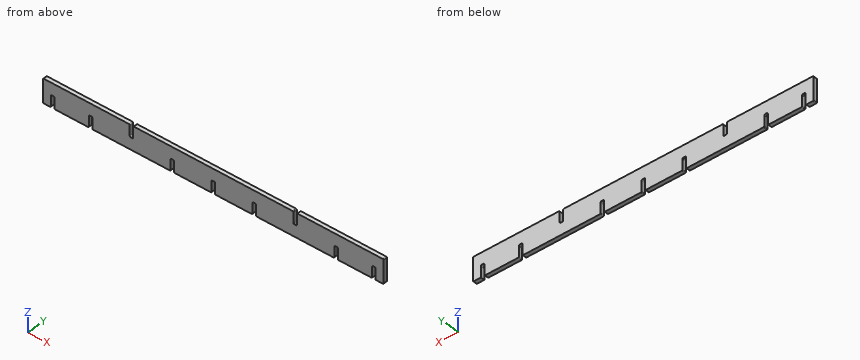
Autodesk Inventor part; units mm, degrees
ref_plane "YZ Plane" through (0, 0, 0) normal (1, 0, 0) x (0, 1, 0)
ref_plane "XZ Plane" through (0, 0, 0) normal (0, 1, 0) x (-1, 0, 0)
ref_plane "XY Plane" through (0, 0, 0) normal (0, 0, 1) x (1, 0, 0)
sketch "Sketch1" plane through (0, 0, 0) normal (0, 1, 0) x (-1, 0, 0)
  line L0 (0, 0) -> (435, 0)
  line L1 (435, 0) -> (435, -30)
  line L2 (435, -30) -> (0, -30)
  line L3 (0, -30) -> (0, 0)
  dimension "d0" = 435
  dimension "d1" = 30
extrude "Extrusion1" add sketch "Sketch1" along normal blind 5
sketch "Sketch2" plane through (0, 5, 0) normal (0, 1, 0) x (1, 0, 0)
  line L0 (0, 30) -> (-435, 30)
  line L1 (-435, 30) -> (-425, 30)
  line L2 (-425, 30) -> (-420.5, 30)
  line L3 (-420.5, 30) -> (-420.5, 15)
  line L4 (-420.5, 15) -> (-425, 15)
  line L5 (-425, 15) -> (-425, 30)
  line L6 (-420.5, 30) -> (-219.75, 30)
  line L7 (-219.75, 30) -> (-215.25, 30)
  line L8 (-215.25, 30) -> (-215.25, 15)
  line L9 (-215.25, 15) -> (-219.75, 15)
  line L10 (-219.75, 15) -> (-219.75, 30)
  line L11 (-215.25, 30) -> (-14.5, 30)
  line L12 (-14.5, 30) -> (-10, 30)
  line L13 (-10, 30) -> (-10, 15)
  line L14 (-10, 15) -> (-14.5, 15)
  line L15 (-14.5, 15) -> (-14.5, 30)
  point P0 (0, 0)
  dimension "d4" = 10
  dimension "d5" = 4.5
  dimension "d6" = 15
  dimension "d7" = 200.75
  dimension "d8" = 4.5
  dimension "d9" = 15
  dimension "d10" = 200.75
  dimension "d11" = 4.5
  dimension "d12" = 15
extrude "Extrusion2" cut sketch "Sketch2" against normal blind 5
sketch "Sketch6" plane through (0, 5, 0) normal (0, 1, 0) x (1, 0, 0)
  line L0 (-14.5, 30) -> (-14.5, 15)
  line L1 (-14.5, 15) -> (-58.5, 15)
  line L2 (-14.5, 30) -> (-215.25, 30)
  line L3 (-58.5, 15) -> (-63, 15)
  line L4 (-63, 15) -> (-63, 30)
  line L5 (-63, 30) -> (-58.5, 30)
  line L6 (-58.5, 30) -> (-58.5, 15)
  line L7 (-63, 15) -> (-110.75, 15)
  line L8 (-110.75, 15) -> (-115.25, 15)
  line L9 (-115.25, 15) -> (-115.25, 30)
  line L10 (-115.25, 30) -> (-110.75, 30)
  line L11 (-110.75, 30) -> (-110.75, 15)
  line L12 (-115.25, 15) -> (-163, 15)
  line L13 (-163, 15) -> (-167.5, 15)
  line L14 (-167.5, 15) -> (-167.5, 30)
  line L15 (-167.5, 30) -> (-163, 30)
  line L16 (-163, 30) -> (-163, 15)
  line L17 (-435, 0) -> (0, 0)
  line L18 (-217.5, 0) -> (-217.5, 47.2454)
  line L19 (-376.5, 15) -> (-372, 15)
  line L20 (-372, 15) -> (-372, 30)
  line L21 (-372, 30) -> (-376.5, 30)
  line L22 (-376.5, 30) -> (-376.5, 15)
  line L23 (-372, 15) -> (-324.25, 15)
  line L24 (-324.25, 15) -> (-319.75, 15)
  line L25 (-319.75, 15) -> (-319.75, 30)
  line L26 (-319.75, 30) -> (-324.25, 30)
  line L27 (-324.25, 30) -> (-324.25, 15)
  line L28 (-319.75, 15) -> (-272, 15)
  line L29 (-272, 15) -> (-267.5, 15)
  line L30 (-267.5, 15) -> (-267.5, 30)
  line L31 (-267.5, 30) -> (-272, 30)
  line L32 (-272, 30) -> (-272, 15)
  line L33 (-110.75, 15) -> (-115.25, 15)
  line L34 (-115.25, 15) -> (-115.25, 0)
  line L35 (-115.25, 0) -> (-110.75, 0)
  line L36 (-110.75, 0) -> (-110.75, 15)
  line L37 (-319.75, 15) -> (-324.25, 15)
  line L38 (-324.25, 15) -> (-324.25, 0)
  line L39 (-324.25, 0) -> (-319.75, 0)
  line L40 (-319.75, 0) -> (-319.75, 15)
  dimension "d40" = 44
  dimension "d41" = 4.5
  dimension "d42" = 47.75
  dimension "d43" = 4.5
  dimension "d44" = 47.75
  dimension "d45" = 4.5
  dimension "d48" = 15
  dimension "d49" = 4.5
  dimension "d50" = 106.75
extrude "Extrusion6" cut sketch "Sketch6" against normal blind 5 contours L19 L22 L21 L20 | L32 L31 L30 L29 | L17 L38 L24 L40 | L6 L3 L4 L2 | L36 L17 L34 L8 | L16 L13 L14 L2
fillet "Fillet2" radius 1 39 edges at (0, 2.5, -30) (-10, 2.5, -15) (-14.5, 2.5, -15) (-14.5, 2.5, -30) (0, 2.5, 0) (-110.75, 2.5, 0) (-115.25, 2.5, 0) (-115.25, 2.5, -15) (-110.75, 2.5, -15) (-63, 2.5, -15) (-58.5, 2.5, -15) (-58.5, 2.5, -30) (-63, 2.5, -30) (-163, 2.5, -15) (-167.5, 2.5, -15) (-163, 2.5, -30) (-167.5, 2.5, -30) (-219.75, 2.5, -30) (-215.25, 2.5, -30) (-215.25, 2.5, -15) (-219.75, 2.5, -15) (-267.5, 2.5, -15) (-272, 2.5, -15) (-272, 2.5, -30) (-267.5, 2.5, -30) (-319.75, 2.5, 0) (-324.25, 2.5, 0) (-324.25, 2.5, -15) (-319.75, 2.5, -15) (-376.5, 2.5, -30) (-376.5, 2.5, -15) (-372, 2.5, -15) (-372, 2.5, -30) (-420.5, 2.5, -30) (-425, 2.5, -30) (-420.5, 2.5, -15) (-425, 2.5, -15) (-435, 2.5, 0) (-435, 2.5, -30)
properties part number "slats" material "Foam Core Board"
Source: CAD feature listing. Evaluate the final solid. Frame: model axes, mm. Round coordinates to 2 decimals unless told otherwise and drop trailing zeros.
(1) Contact query for flat-ended pins moving along their axis: pin 1 Ø1.2 at (x, y) = (-322, 3) entering from +Z; pin 2 Ø3 at (x, y) = (-269.5, 3) entering from -Z; pin 3 Ø3 at (x, y) = (-112.5, 3) entering from +Z; pin 4 Ø3 at (x, z) = (-391.5, -9) entering from -Y. Output: stop coordinate, or through.
From the geometry:
pin 1: stops at z = -15
pin 2: stops at z = -15.13
pin 3: stops at z = -14.66
pin 4: stops at y = 0
(2) Material intervals for probe 1 along X at (y, z) = (4.05, -3.5), sorted ascending.
From the geometry:
probe 1: x = -435 to -324.25, -319.75 to -115.25, -110.75 to 0
(3) Section query A-A (z = -24.5). Give the number of separate pieces and of enclosed holes in the cut face, and give its area (3 significant figures).
From the geometry:
separate pieces: 8
enclosed holes: 0
area: 2,020 mm2
